For this review, take the finished solid that the model builds, in its own axes (mm). A direction names the side the tool comes from. Give positions to 0.01 mm unless a question says otherwise; leave off trailing zeros. Write each loop counter-clockwise with the first axis right and the second up, starting at its lowest first coordinate (ties: lowest second). Pieces come first, ordered by that corner, then holes.
1) Draft analysis for pull direction X (two halves, no side actions). For faces 1 (the face through (-18.44, -22.44, 0.99)), 2 (the face through (-10.627, -28.042, 0.986)), 3 (the face through (-9.8, -13.9, 1)), 4 (the face through (1.295, -16.154, 0.986)), state which applies: pulls with the +X half, pulls with the -X half, needs draft (parallel to the pull), parting line crosses it, or undercut.
2) Machinability: for faces 5 (the face through (0, -5, 1)), 6 (the face through (-23.53, -13.06, 1.01)), 7 (the face through (-13.56, -19.9, 0.99)), 8 (the face through (-9, 0, 1)), 9 (the face through (-17, -5, 1)), which of the approach directions +Z, -Z, +X, -X, +Y, -Y give a long, thin tool a straight path to every point of the face, cutting with its end or side? Answer none if there is none.
3) We need section B-B on x = -3.5. Give the boundary of the cut face in (y, z).
4) We need section C-C on y = -20.5. Give the boundary of the cut face in (x, z), and give its area (3 significant figures).
5) We need section A-A on y = -5. Give the boundary of the cut face in (x, z).
6) Wall thickness on line 1 along Y through (x, z) = (-3.5, 1.6); line 2 along X through (y, z) = (-15, 1.1); line 3 along Y through (x, z) = (-4.25, 0.85): over which ranges is each line inside the solid? List them lowest first.
7) For P1, Ø1, axis at y = -4, z = 1, coming from the -X side; P2, Ø1, axis at y = -6, z = 0.5, coming from the +X side; P3, Ø1, axis at y = -21, z = 1, coming from the +X side, all flat-tipped, find the tip position at first contact; note any pin that passes through.
8) We need section D-D on z = 0.85. Give the boundary of the cut face in (x, y).
from build123d import *

# Parameters (mm, degrees)
SKETCH_1_R          = 1.5
EXTRUDE_1_DEPTH     = 2
SKETCH_2_W          = 2
SKETCH_2_H          = 22.232050807
EXTRUDE_2_DEPTH     = 8
CUT_EXTRUDE_1_DEPTH = 5
FILLET_1_R          = 1


with BuildPart() as part:
    # 草图1 → 凸台-拉伸1 (new body)
    with BuildSketch(Plane.XY):
        Polygon((-17, 0), (0, 0), (0, -10), (2.776279442, -23.191342951), (-5.883974596, -28.191342951), (-17, -8.937822174), align=None)
        with Locations((-3.303847577, -22.660254038)):
            Circle(SKETCH_1_R, mode=Mode.SUBTRACT)
        with Locations((-13.5, -5)):
            Circle(SKETCH_1_R, mode=Mode.SUBTRACT)
        with Locations((-8.303847577, -14)):
            Circle(SKETCH_1_R, mode=Mode.SUBTRACT)
        with Locations((-3.5, -5)):
            Circle(SKETCH_1_R, mode=Mode.SUBTRACT)
    extrude(amount=EXTRUDE_1_DEPTH)

    # 草图2 → 凸台-拉伸2 (add)
    with BuildSketch(Plane(origin=(-16.620190528, -9.595671476, 0), x_dir=(0, 0, 1), z_dir=(-0.866025404, -0.5, 0))):
        with Locations((1, -10.356406461)):
            Rectangle(SKETCH_2_W, SKETCH_2_H)
    extrude(amount=EXTRUDE_2_DEPTH)

    # 草图3 → 切除-拉伸1 (cut)
    with BuildSketch(Plane(origin=(0, 0, 0), x_dir=(-1, 0, 0), z_dir=(0, 0, -1))):
        with BuildLine():
            Line((10.049038106, -25.977241336), (17.165063509, -13.651923789))
            ThreePointArc((17.165063509, -13.651923789), (19.214101615, -13.102885683), (19.763139721, -15.151923789))
            Line((19.763139721, -15.151923789), (12.647114317, -27.477241336))
            ThreePointArc((12.647114317, -27.477241336), (10.598076211, -28.026279442), (10.049038106, -25.977241336))
        make_face()
    extrude(amount=-CUT_EXTRUDE_1_DEPTH, mode=Mode.SUBTRACT)

    # 圆角1
    fillet_1_edges = [part.edges().sort_by_distance(p)[0] for p in [
        (2.776279442, -23.191342951, 1),
        (-17, 0, 1),
        (0, 0, 1),
        (-23.92820323, -12.937822174, 1),
        (-12.812177826, -32.191342951, 1),
    ]]
    fillet(fillet_1_edges, radius=FILLET_1_R)


solid = part.part
Results list:
1. face 1: pulls with the -X half
1. face 2: undercut
1. face 3: undercut
1. face 4: pulls with the +X half
2. face 5: +Z, -Z, +X, +Y
2. face 6: +Z, -Z, -X
2. face 7: +Z, -Z
2. face 8: +Z, -Z, +X, -X, +Y
2. face 9: +Z, -Z, -X, +Y
3. outline: (-26.81, 0) - (-24.15, 0) - (-24.15, 2) - (-26.81, 2) - close; (-21.17, 0) - (-6.5, 0) - (-6.5, 2) - (-21.17, 2) - close; (-3.5, 0) - (0, 0) - (0, 2) - (-3.5, 2) - close
4. outline: (-19.56, 0) - (-16.68, 0) - (-16.68, 2) - (-19.56, 2) - close; (-13.21, 0) - (2.21, 0) - (2.21, 2) - (-13.21, 2) - close
4. area: 36.6 mm2
5. outline: (-17, 0) - (-15, 0) - (-15, 2) - (-17, 2) - close; (-12, 0) - (-5, 0) - (-5, 2) - (-12, 2) - close; (-2, 0) - (0, 0) - (0, 2) - (-2, 2) - close
6. line 1: y = -26.81 to -24.15, -21.17 to -6.5, -3.5 to 0
6. line 2: x = -22.74 to -19.84, -16.39 to -9.42, -7.19 to 1.05
6. line 3: y = -27.25 to -23.82, -21.5 to -6.3, -3.7 to 0
7. P1: stops at x = -17
7. P2: stops at x = 0
7. P3: stops at x = 2.42
8. outline: (-23.43, -13.8) - (-13.31, -31.33) arc R1 ccw to (-11.95, -31.69) - (2.15, -23.55) arc R1 ccw to (2.63, -22.48) - (0, -10) - (0, -1) arc R1 ccw to (-1, 0) - (-16, 0) arc R1 ccw to (-17, -1) - (-17, -8.94) - (-23.06, -12.44) arc R1 ccw to start; hole (-19.76, -15.15) - (-12.65, -27.48) arc R1.5 ccw to (-10.05, -25.98) - (-17.17, -13.65) arc R1.5 ccw to start; hole circle Ø3 at (-13.5, -5); hole circle Ø3 at (-8.3, -14); hole circle Ø3 at (-3.5, -5); hole circle Ø3 at (-3.3, -22.66)
